The model under review builds one solid part; all positions refer to its coordinate system, in mm. Face numbers are marked on the shaded views. A direction names the side the tool comes from. Round coordinates to 2 decimals unless told otherwise and drop trailing zeros. Write each loop counter-clockwise with the first axis right and the second up, starting at its lowest first coordinate (ties: lowest second). Pieces come first, ordered by that corner, then holes. Notation, with made-up numbers: (-1.75, 31) - (24.25, 31) arc R30 ccw to (24.25, 65) - close; hole circle Ø3 at (7, -31.75). An arc over 180 degrees is marked (long way). Write each question's results on one line, items separated by ' | '.
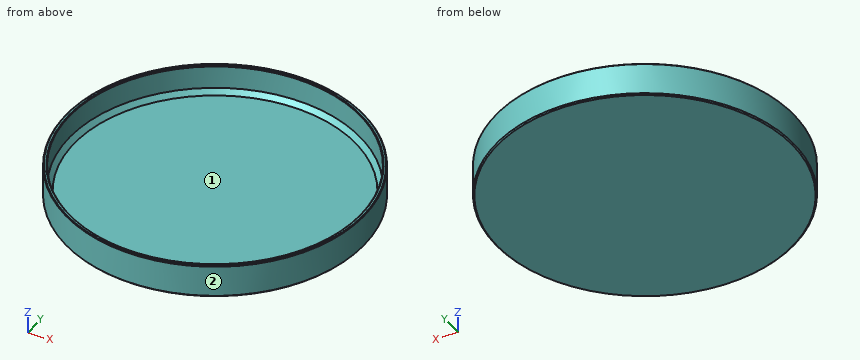
```python
from build123d import *

# Parameters (mm, degrees)
F0_R     = 63.1
F0_R_2   = 61.6
F1_DEPTH = 2
F2_DEPTH = 14
F3_SIZE  = 0.5
F4_SIZE  = 2
F5_SIZE  = 0.3


# Not quite as in the source:
# - a feature names something its author has since deleted; it is built from what else it names


with BuildPart() as f1:
    # F0 (on Top) → F1 (new body)
    with BuildSketch(Plane.XY):
        Circle(F0_R)
        Circle(F0_R_2, mode=Mode.SUBTRACT)
        Circle(F0_R_2)
    extrude(amount=F1_DEPTH)

    # F0 (on Top) → F2 (join)
    with BuildSketch(Plane.XY):
        Circle(F0_R)
        Circle(F0_R_2, mode=Mode.SUBTRACT)
    extrude(amount=F2_DEPTH)

    # F3
    f3_edges = [f1.edges().sort_by_distance(p)[0] for p in [
        (-63.1, 0, 0),
    ]]
    chamfer(f3_edges, length=F3_SIZE)

    # F4
    f4_edges = [f1.edges().sort_by_distance(p)[0] for p in [
        (-61.6, 0, 2),
    ]]
    chamfer(f4_edges, length=F4_SIZE)

    # F5
    f5_edges = [f1.edges().sort_by_distance(p)[0] for p in [
        (-63.1, 0, 14),
        (-61.6, 0, 14),
    ]]
    chamfer(f5_edges, length=F5_SIZE)


solid = f1.part
```
Q1. We need section A-A (y = 0). State the section outline as (x, z) points, plus the area to 3 significant figures.
Evaluation:
outline: (-63.1, 0.5) - (-62.6, 0) - (62.6, 0) - (63.1, 0.5) - (63.1, 13.7) - (62.8, 14) - (61.9, 14) - (61.6, 13.7) - (61.6, 4) - (59.6, 2) - (-59.6, 2) - (-61.6, 4) - (-61.6, 13.7) - (-61.9, 14) - (-62.8, 14) - (-63.1, 13.7) - close | area: 292 mm^2
Q2. Tool access review of the marked faces 1 and 2: name each direction out of +Z, -Z, +X, -X, +Y, -Y from which nothing blocks a thin tool from reaching the whole face with its end or side.
Evaluation:
face 1: +Z | face 2: +Z, -Z
Q3. We need section C-C (z = 6.5). State the section outline as (x, y) points, plus the area to 3 significant figures.
Evaluation:
outline: circle Ø126.2 at (0, 0); hole circle Ø123.2 at (0, 0) | area: 588 mm^2
Q4. For probe 1 along Y at (x, z) = (0, 6.5); probe 2 along Z at (x, y) = (11, -42.5); probe 3 along Y at (x, z) = (49.5, 12.5), list the stretches that pass through material, from the lowest coordinate up.
Evaluation:
probe 1: y = -63.1 to -61.6, 61.6 to 63.1 | probe 2: z = 0 to 2 | probe 3: y = -39.13 to -36.66, 36.66 to 39.13
Q5. Insertion check: P1, Ø2, axis at x = 30.5, z = 12, coming from the -Y side; P2, Ø5, axis at x = 34.5, y = 31.5, coming from the +Z side; P3, Ø3, axis at y = 17.5, z = 3.5, coming from the -X side. Each pin has a flat end and moves straight along its axis. Give the tip position at first contact, or say it passes through.
Evaluation:
P1: stops at y = -55.78 | P2: stops at z = 2 | P3: stops at x = -61.04
